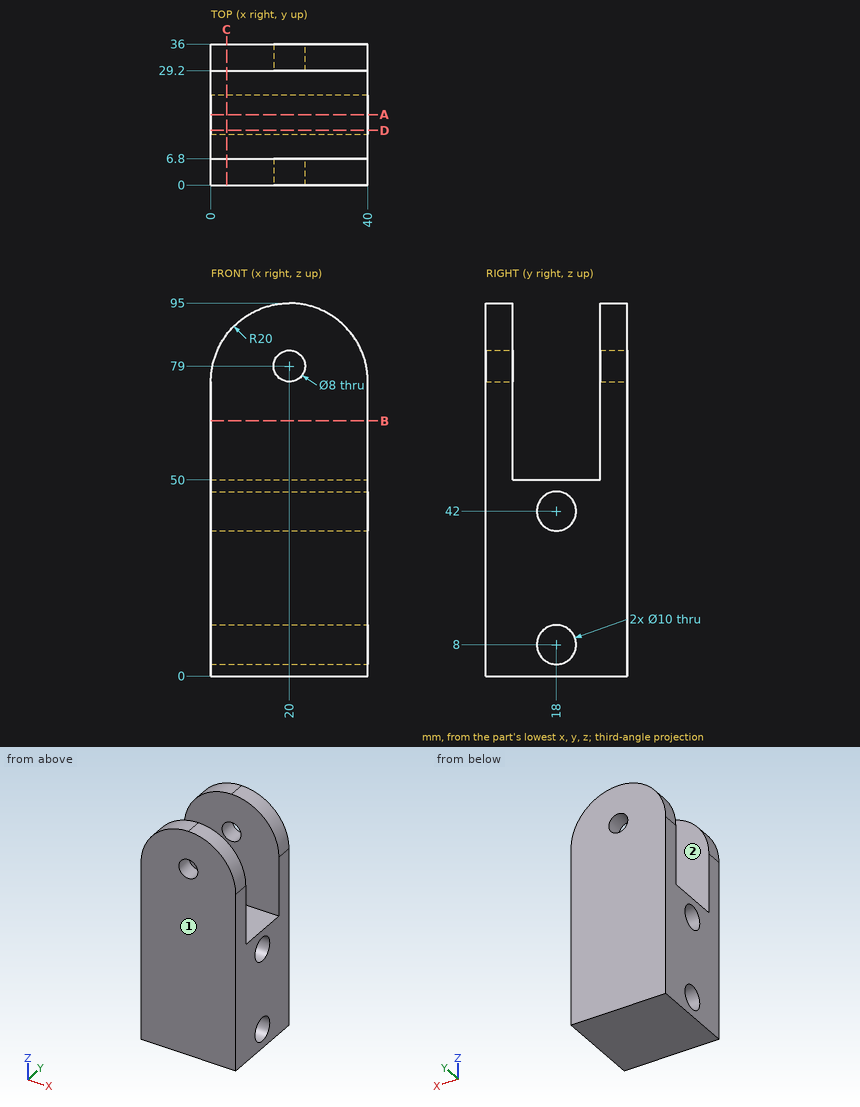
Could you check a few things on this drawing? It's one solid part, dimensions in mm from its lowest x, y, z. A direction names the side the tool comes from. Round coordinates to 2 decimals unless told otherwise and drop trailing zeros. Loops run counter-clockwise (first coordinate to the right, second up) from the corner with the lowest first, then second, coordinate; pieces in that order, holes last.
Q1. For P1, Ø3, axis at y = 6, z = 77, coming from the +X side, with a flat end and sliding along its axis, tell me the tip position at first contact or that it passes through.
Q2. Please list where these lines run through material, in increasing order: L1, parallel to Z at x = 21, y = 18; L2, parallel to Z at x = 20, y = 31; L3, parallel to Y at x = 9, z = 77.5.
Q3. On a 3-axis mill with a long thin cutter (end or side, diameter ignored), from which of +Z, -Z, +X, -X, +Y, -Y can I reach the whole of each face in a straight line? I mean the marked faces 1 and 2. Say none if no direction works.
Q4. I want a section at B-B (z = 65). Write out the boundary of the cut face in (x, y), and give its area (3 significant figures).
Q5. I want a section at A-A (y = 18). Write out the boundary of the cut face in (x, z), and give its area (3 significant figures).
Q6. I want a section at D-D (y = 14). Write out the boundary of the cut face in (x, z).
Q7. I want a section at C-C (x = 4). Write out the boundary of the cut face in (y, z), and give its area (3 significant figures).
Answer below:
1. P1: stops at x = 39.99
2. L1: z = 0 to 3, 13 to 37, 47 to 50
2. L2: z = 0 to 75, 83 to 95
2. L3: y = 0 to 6.8, 29.2 to 36
3. face 1: +Z, -Z, +X, -X, -Y
3. face 2: +Z, +X, -X
4. outline: (0, 0) - (40, 0) - (40, 6.8) - (0, 6.8) - close; (0, 29.2) - (40, 29.2) - (40, 36) - (0, 36) - close
4. area: 544 mm2
5. outline: (0, 0) - (40, 0) - (40, 3) - (0, 3) - close; (0, 13) - (40, 13) - (40, 37) - (0, 37) - close; (0, 47) - (40, 47) - (40, 50) - (0, 50) - close
5. area: 1,200 mm2
6. outline: (0, 0) - (40, 0) - (40, 5) - (0, 5) - close; (0, 11) - (40, 11) - (40, 39) - (0, 39) - close; (0, 45) - (40, 45) - (40, 50) - (0, 50) - close
7. outline: (0, 0) - (36, 0) - (36, 87) - (29.2, 87) - (29.2, 50) - (6.8, 50) - (6.8, 87) - (0, 87) - close; hole circle Ø10 at (18, 8); hole circle Ø10 at (18, 42)
7. area: 2,150 mm2
